Geometry check sheet. Reference: drawing and pictorial views, mm from the part's lowest x, y, z. Round coordinates to 2 decimals unless told otherwise and drop trailing zeros. Write each loop counter-clockwise with the first axis right and the second up, starting at its lowest first coordinate (ties: lowest second). Pieces come first, ordered by that corner, then holes. Notation, with made-up numbers: M -8.75,51 L 38.25,51 A27 ccw 38.25,78 Z; hole C 42,4 d4. An arc over 180 degrees is marked long. One line per item, written item: value. Start each with the question number.
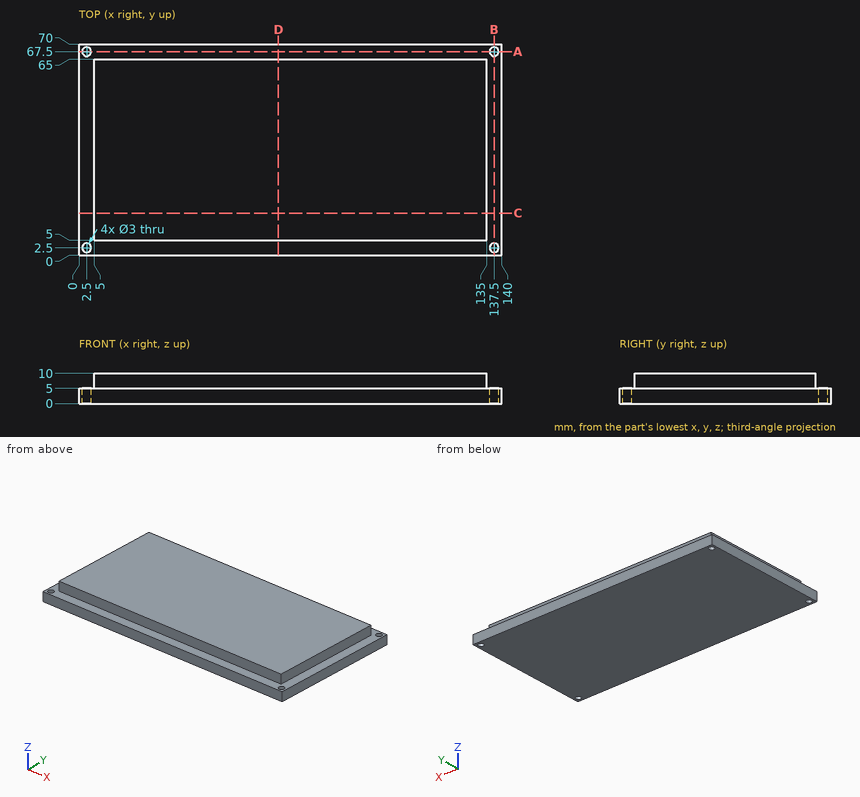
1) Gauge pin test, flat ends, axial feed: pin 1 Ø12 at (x, y) = (46, 60.5) entering from -Z; pin 2 Ø5 at (x, y) = (2.5, 67.5) entering from +Z; pin 3 Ø1.8 at (x, y) = (137.5, 67.5) entering from +Z; pin 4 Ø2.5 at (x, z) = (98.5, 8) entering from +Y. Record the tip position at first contact, or that the pin passes through.
2) Cross-section at A-A (y = 67.5). Record the boundary of the cut face in (x, z).
3) Cross-section at B-B (x = 137.5). Record the boundary of the cut face in (y, z).
4) Cross-section at C-C (y = 14). Record the boundary of the cut face in (x, z), then the cut area to 3 significant figures.
5) Cross-section at D-D (x = 66). Record the boundary of the cut face in (y, z), then the cut area to 3 significant figures.
6) Thickness scan on line 1 (X direction, y = 67.5, z = 2); line 2 (Y direction, x = 2.5, z = 2.3); line 3 (X direction, y = 43, z = 5.75). Record the ranges inside material, lowest first.
Results below:
1. pin 1: stops at z = 0
1. pin 2: stops at z = 5
1. pin 3: passes through
1. pin 4: stops at y = 65
2. outline: M 0,0 L 1,0 L 1,5 L 0,5 Z; M 4,0 L 136,0 L 136,5 L 4,5 Z; M 139,0 L 140,0 L 140,5 L 139,5 Z
3. outline: M 0,0 L 1,0 L 1,5 L 0,5 Z; M 4,0 L 66,0 L 66,5 L 4,5 Z; M 69,0 L 70,0 L 70,5 L 69,5 Z
4. outline: M 0,0 L 140,0 L 140,5 L 135,5 L 135,10 L 5,10 L 5,5 L 0,5 Z
4. area: 1,350 mm²
5. outline: M 0,0 L 70,0 L 70,5 L 65,5 L 65,10 L 5,10 L 5,5 L 0,5 Z
5. area: 650 mm²
6. line 1: x = 0 to 1, 4 to 136, 139 to 140
6. line 2: y = 0 to 1, 4 to 66, 69 to 70
6. line 3: x = 5 to 135
